Drawing for the job (mm, zero at the part's lowest x, y, z). Round coordinates to 2 decimals unless told otherwise and drop trailing zeros. Write each loop counter-clockwise with the first axis right and the second up, starting at its lowest first coordinate (ties: lowest second). Pieces come first, ordered by that corner, then holes. Notation, with made-up numbers: M 76,80.25 L 106,80.25 A20 cw 106,94.25 Z; hole C 87,68 d10. An arc over 180 degrees is marked long. Use a Markdown table: item, result. Add a question column.
1) Slice it at A-A on x = 45. Write the cut outline in (y, z), plus the area to 3 significant figures.
2) Wall check: probe 1 along Y at (x, z) = (42.5, 2). Give the ranges that are in metal, low to high.
3) Drop flat-ended pins along their axis: P1, Ø1.5, axis at y = 101.5, z = 2, coming from the +X side; P2, Ø1.5, axis at x = 46, z = 2, coming from the +Y side. Give the stop position or say it passes through.
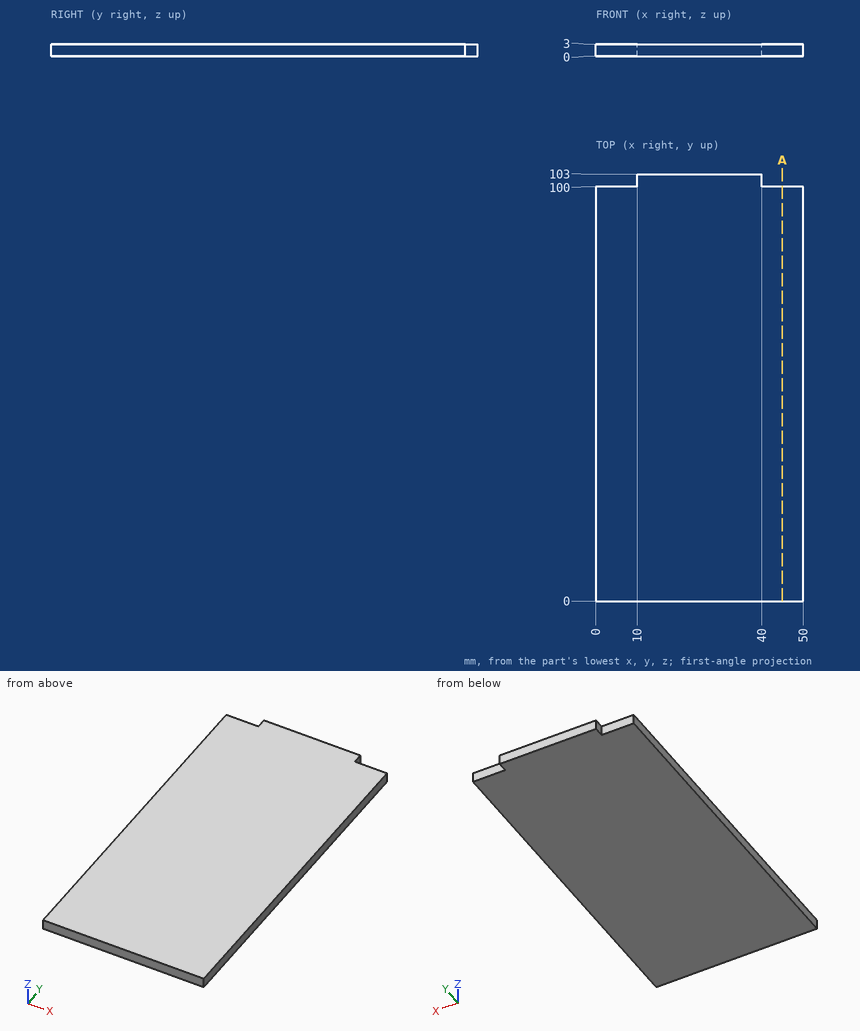
Entries:
| question | item | result |
|---|---|---|
| 1 | outline | M 0,0 L 100,0 L 100,3 L 0,3 Z |
| 1 | area | 300 mm^2 |
| 2 | probe 1 | y = 0 to 100 |
| 3 | P1 | stops at x = 40 |
| 3 | P2 | stops at y = 100 |
